Read the model definition and answer for the solid it produces. Units are mm, in the model's axes. Give positions to 0.01 mm unless a question says otherwise; leave off trailing zeros. Order: outer loops, then holes, each group sorted by start corner. A loop starts at its lowest first (then second) coordinate and runs counter-clockwise, first axis right, second up. Notation, with made-up numbers: (16, 11) - (40, 11) arc R17 ccw to (40, 43) - close; hole circle Ø11 at (-17.75, -4). An arc over 180 degrees is marked (long way). Return JSON: item names as keys, results as strings.
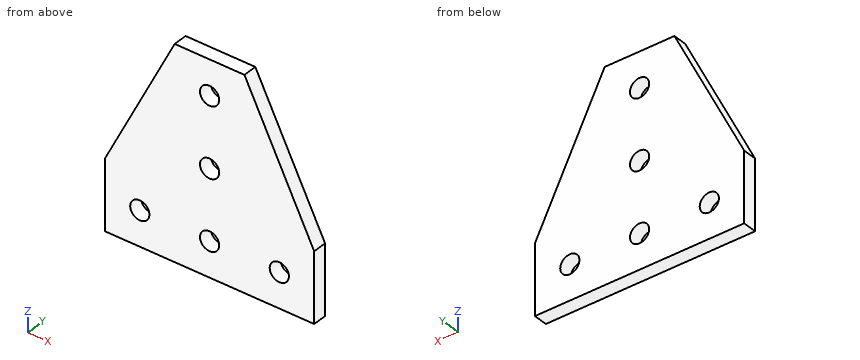
```python
from build123d import *

# Parameters (mm, degrees)
F0_R     = 2.75
F1_DEPTH = 4


with BuildPart() as f1:
    # F0 (on Front) → F1 (new body)
    with BuildSketch(Plane.XZ):
        Polygon((-30, -10), (-30, -30), (30, -30), (30, -10), (10, 30), (-10, 30), align=None)
        with Locations((-20, -20)):
            Circle(F0_R, mode=Mode.SUBTRACT)
        with Locations((0, -20)):
            Circle(F0_R, mode=Mode.SUBTRACT)
        with Locations((20, -20)):
            Circle(F0_R, mode=Mode.SUBTRACT)
        Circle(F0_R, mode=Mode.SUBTRACT)
        with Locations((0, 20)):
            Circle(F0_R, mode=Mode.SUBTRACT)
    extrude(amount=F1_DEPTH)


solid = f1.part
```
Q1. A cutting plane is placed at B-B (z = 0). Write down the section's boundary in (x, y).
Values:
{"outline": "(-25, -4) - (-2.75, -4) - (-2.75, 0) - (-25, 0) - close; (2.75, -4) - (25, -4) - (25, 0) - (2.75, 0) - close"}
Q2. Given pin 1 (3.5 mm diameter, centred on x = 20, z = -20, fed in from -Y); pin 2 (2 mm diameter, centred on y = -1, z = 17, fed in from -X), each flat-ended and moving along its own axis, determine where each tip first touches the part or whether it passes through.
Values:
{"pin 1": "passes through", "pin 2": "stops at x = -17"}
Q3. A cutting plane is placed at A-A (x = 0). Write down the section's boundary in (y, z).
Values:
{"outline": "(-4, -30) - (0, -30) - (0, -22.75) - (-4, -22.75) - close; (-4, -17.25) - (0, -17.25) - (0, -2.75) - (-4, -2.75) - close; (-4, 2.75) - (0, 2.75) - (0, 17.25) - (-4, 17.25) - close; (-4, 22.75) - (0, 22.75) - (0, 30) - (-4, 30) - close"}
Q4. A cutting plane is placed at D-D (y = -3.15). Write down the section's boundary in (x, z), and give its area (3 significant figures).
Values:
{"outline": "(-30, -30) - (30, -30) - (30, -10) - (10, 30) - (-10, 30) - (-30, -10) - close; hole circle Ø5.5 at (-20, -20); hole circle Ø5.5 at (0, -20); hole circle Ø5.5 at (0, 0); hole circle Ø5.5 at (0, 20); hole circle Ø5.5 at (20, -20)", "area": "2,680 mm²"}
Q5. Consider L1, parallel to Z at x = 0, y = -0.85; L2, parallel to Z at x = 1, y = -1.6; L3, parallel to Z at x = 20, y = -2.3. Determine where each line is inside the solid, lowest interval first.
Values:
{"L1": "z = -30 to -22.75, -17.25 to -2.75, 2.75 to 17.25, 22.75 to 30", "L2": "z = -30 to -22.56, -17.44 to -2.56, 2.56 to 17.44, 22.56 to 30", "L3": "z = -30 to -22.75, -17.25 to 10"}
Q6. A cutting plane is placed at C-C (x = 20). Write down the section's boundary in (y, z).
Values:
{"outline": "(-4, -30) - (0, -30) - (0, -22.75) - (-4, -22.75) - close; (-4, -17.25) - (0, -17.25) - (0, 10) - (-4, 10) - close"}
